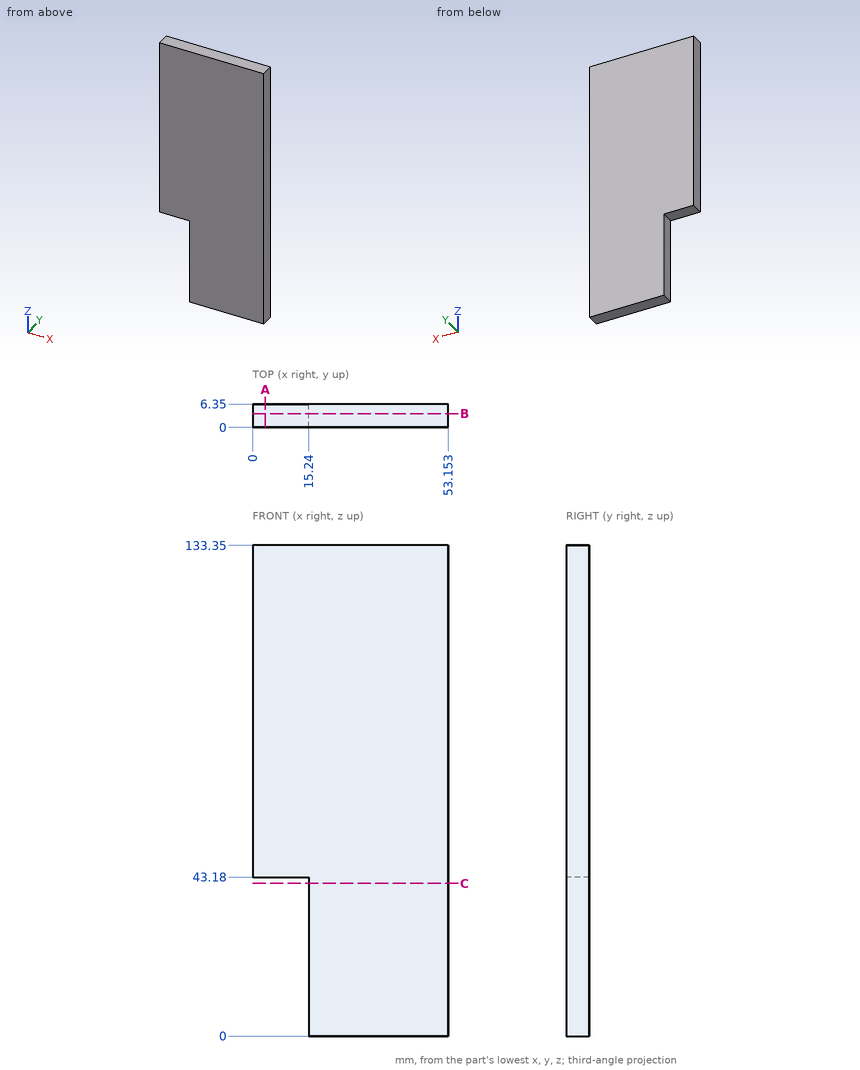
For this review, use the dimensioned drawing (mm, ordinates from the lowest corner) and the shaded views. Round coordinates to 2 decimals unless told otherwise and drop trailing zeros. Write each loop counter-clockwise with the first axis right and the second up, starting at its lowest first coordinate (ties: lowest second). Pieces come first, ordered by that corner, then holes. Notation, with made-up numbers: (-31, 82) -> (18, 82) arc R18 cw to (18, 103) -> close; hole circle Ø2 at (23.25, 61.5). An arc over 180 degrees is marked (long way). Answer in a Markdown table with one row per item.
Q1. Clearance check with a flat-ended pin moving along its axis: pin 1 Ø1.9 at (y, z) = (4.5, 22.5) entering from -X. State where the tip first meets the part, or that it passes through.
The answers:
| item | result |
|---|---|
| pin 1 | x = 15.24 |
Q2. Take a section at B-B, the plane y = 3.75. State the section outline as (x, z) points.
The answers:
| item | result |
|---|---|
| outline | (0, 43.18) -> (15.24, 43.18) -> (15.24, 0) -> (53.15, 0) -> (53.15, 133.35) -> (0, 133.35) -> close |
Q3. Take a section at A-A, the plane x = 3.5. State the section outline as (y, z) points.
The answers:
| item | result |
|---|---|
| outline | (0, 43.18) -> (6.35, 43.18) -> (6.35, 133.35) -> (0, 133.35) -> close |
Q4. Take a section at C-C, the plane z = 41.5. State the section outline as (x, y) points.
The answers:
| item | result |
|---|---|
| outline | (15.24, 0) -> (53.15, 0) -> (53.15, 6.35) -> (15.24, 6.35) -> close |
Q5. To check wall thickness, follow L1, parallel to X at y = 5.25, z = 41; L2, parallel to Z at x = 6.5, y = 5.25. State the ranges of each line that lie inside material, in increasing order. Write a range as [from, to].
The answers:
| item | result |
|---|---|
| L1 | [15.24, 53.15] |
| L2 | [43.18, 133.35] |
